from build123d import *

# Parameters (mm, degrees)
SKETCH001_W   = 13.6
SKETCH001_H   = 42.6
SKETCH001_W_2 = 11
SKETCH001_H_2 = 40
PAD_DEPTH     = 20
SKETCH002_R   = 20
SKETCH005_R   = 5.8
PAD001_DEPTH  = 4


with BuildPart() as part:
    # Sketch001 → Pad (new body)
    with BuildSketch(Plane.XY):
        Rectangle(SKETCH001_W, SKETCH001_H)
        Rectangle(SKETCH001_W_2, SKETCH001_H_2, mode=Mode.SUBTRACT)
    extrude(amount=PAD_DEPTH)

    # Sketch002 → Groove (revolve, cut)
    with BuildSketch(Plane(origin=(-6.8, 0, 0), x_dir=(0, -1, 0), z_dir=(-1, 0, 0))):
        with Locations((0, 20)):
            Circle(SKETCH002_R)
    revolve(axis=Axis((-6.8, 20, 40), (0, -1, 0)), mode=Mode.SUBTRACT)

    # Sketch005 → Pad001 (new body)
    with BuildSketch(Plane(origin=(0, 0, 0), x_dir=(1, 0, 0), z_dir=(0, 0, -1))):
        with BuildLine():
            Line((-6.8, 21.3), (6.8, 21.3))
            Line((6.8, 21.3), (6.8, -35.514262))
            ThreePointArc((-6.8, -35.514262), (0, -39.3), (6.8, -35.514262))
            Line((-6.8, -35.514262), (-6.8, 21.3))
        make_face()
        with Locations((-0.017483, -31.296471)):
            Circle(SKETCH005_R, mode=Mode.SUBTRACT)
    extrude(amount=PAD001_DEPTH)


solid = part.part
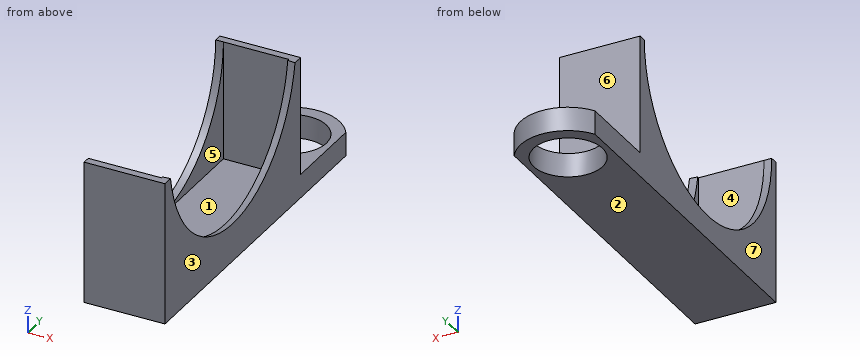
Source: CAD feature listing. Evaluate the final solid. Frame: model axes, mm. Face numbers are marked on the shaded views. A direction names the side the tool comes from. Coordinates: 2 decimals unless noted, no trailing zeros. Write each loop counter-clockwise with the first axis right and the second up, starting at its lowest first coordinate (ties: lowest second). Pieces come first, ordered by that corner, then holes. Notation, with made-up numbers: M -7.5,6.5 L 1.5,6.5 A29 cw 1.5,31.5 Z; hole C 67,4 d7. An arc over 180 degrees is marked long. Use a Markdown table: item, result.
1) Section C-C, the plane x = -2.75. Output: boundary loops of the cut face in (y, z), then the cut area to 3 significant figures.
Conclusion:
| item | result |
|---|---|
| outline | M -21.3,-4 L 26.18,-4 L 26.18,0 L 21.3,0 L 21.3,20 L 20,20 L 20,0 L -20,0 L -20,20 L -21.3,20 Z; M 36.41,-4 L 38.81,-4 L 38.81,0 L 36.41,0 Z |
| area | 252 mm^2 |
2) Reachability of the marked faces 5, 6 and 7 from +Z, -Z, +X, -X, +Y, -Y: full face, straight path, thin tool, end or side. Return the list, or none.
Conclusion:
| item | result |
|---|---|
| face 5 | +Z |
| face 6 | +Z, +X, -X, +Y |
| face 7 | +Z, -Z, -X, +Y, -Y |
3) First-contact query: pin 1 Ø4 at (x, y) = (2.5, 32.5) entering from +Z; pin 2 Ø5.5 at (x, z) = (-2, 11.5) entering from +Y; pin 3 Ø3 at (x, y) = (-2, -6.5) entering from +Z. Flat tips, straight axial feed; report the tip coordinate or a pass-through.
Conclusion:
| item | result |
|---|---|
| pin 1 | passes through |
| pin 2 | stops at y = 21.3 |
| pin 3 | stops at z = 0 |
4) Section A-A, the plane x = 1.5. Output: boundary loops of the cut face in (y, z), then the cut area to 3 significant figures.
Conclusion:
| item | result |
|---|---|
| outline | M -21.3,-4 L 25.7,-4 L 25.7,0 L 21.3,0 L 21.3,20 L 20,20 L 20,0 L -20,0 L -20,20 L -21.3,20 Z; M 36.89,-4 L 39.16,-4 L 39.16,0 L 36.89,0 Z |
| area | 249 mm^2 |
5) Mould query, pull axis X, two halves, no side actions, for the marked faces 1, 2, 3 and 4. Classes: pulls with the +X half, pulls with the -X half, needs draft (parallel to the pull), parting line crosses it, or undercut.
Conclusion:
| item | result |
|---|---|
| face 1 | undercut |
| face 2 | needs draft |
| face 3 | pulls with the +X half |
| face 4 | undercut |
6) Ray query, L1, parallel to Y at x = -4.75, z = 8; L2, parallel to X at y = 19, z = 1.75; L3, parallel to Z at x = -5, y = -15. Return the intervals inside material, ascending.
Conclusion:
| item | result |
|---|---|
| L1 | y = -21.3 to -20, 20 to 21.3 |
| L2 | x = -6.8 to -5.5, 5.5 to 6.8 |
| L3 | z = -4 to 0 |
7) Section B-B, the plane y = 27.5. Output: boundary loops of the cut face in (x, z).
Conclusion:
| item | result |
|---|---|
| outline | M -6.8,-4 L -4.4,-4 L -4.4,0 L -6.8,0 Z; M 4.37,-4 L 6.8,-4 L 6.8,0 L 4.37,0 Z |
